```python
from build123d import *

# Parameters (mm, degrees)
SKETCH1_R           = 1.75
BOSS_EXTRUDE1_DEPTH = 5
SKETCH2_R           = 1.75
SKETCH2_R_2         = 6.2
CUT_EXTRUDE1_DEPTH  = 10


with BuildPart() as part:
    # Sketch1 → Boss-Extrude1 (new body)
    # profile 1 of 4: a face of its own
    with BuildSketch(Plane(origin=(0, 0, 0), x_dir=(1, 0, 0), z_dir=(0, 1, 0))):
        Polygon((50, 25), (0, 25), (0, 15), (10, 0), (26, 0), (36, 15), (50, 15), align=None)
        with Locations(Location((13, 5, 0), (0, 0, 270))):
            Circle(SKETCH1_R, mode=Mode.SUBTRACT)
        with Locations(Location((23, 5, 0), (0, 0, 270))):
            Circle(SKETCH1_R, mode=Mode.SUBTRACT)
    # profile 2 of 4: a face of its own
    with BuildSketch(Plane(origin=(0, 0, 0), x_dir=(1, 0, 0), z_dir=(0, 1, 0))):
        Polygon((10, 45), (0, 33.819660113), (0, 25), (50, 25), (50, 35), (36, 35), (26, 45), align=None)
    # profile 3 of 4: a face of its own
    with BuildSketch(Plane(origin=(0, 0, 0), x_dir=(1, 0, 0), z_dir=(0, 1, 0))):
        Polygon((10, 45), (0, 33.819660113), (0, 25), (50, 25), (50, 35), (36, 35), (26, 45), align=None)
    # profile 4 of 4: a face of its own
    with BuildSketch(Plane(origin=(0, 0, 0), x_dir=(1, 0, 0), z_dir=(0, 1, 0))):
        Polygon((10, 45), (0, 33.819660113), (0, 25), (50, 25), (50, 35), (36, 35), (26, 45), align=None)
    extrude(amount=BOSS_EXTRUDE1_DEPTH)

    # Sketch2 → Cut-Extrude1 (cut)
    with BuildSketch(Plane(origin=(0, 0, 0), x_dir=(-1, 0, 0), z_dir=(0, -1, 0))):
        with Locations(Location((-4.8, 24.409830056, 0), (0, 0, 90))):
            Circle(SKETCH2_R)
        with Locations(Location((-32.8, 24.409830056, 0), (0, 0, 90))):
            Circle(SKETCH2_R_2)
    extrude(amount=-CUT_EXTRUDE1_DEPTH, mode=Mode.SUBTRACT)


solid = part.part
```
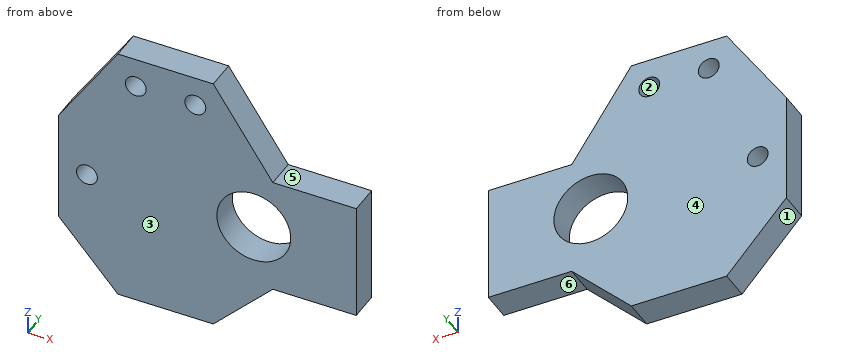
Read the model definition and answer for the solid it produces. Units are mm, in the model's axes. Face numbers are marked on the shaded views. A direction names the side the tool comes from. Coordinates: 2 decimals unless noted, no trailing zeros. Loops run counter-clockwise (first coordinate to the right, second up) from the corner with the lowest first, then second, coordinate; pieces in that order, holes last. Notation, with made-up numbers: (64.5, -39) -> (107.5, -39) arc R25 cw to (107.5, -2) -> close; hole circle Ø7 at (80, -3.5). An arc over 180 degrees is marked (long way). Return JSON: item names as keys, results as strings.
Item 1: For a pull along X with two mould halves and no side action, classify the marked faces 1, 2 and 3 as +X half, -X half, draft (parallel to the pull), parting line (faces both ways), or undercut.
Answers:
{"face 1": "-X half", "face 2": "undercut", "face 3": "draft"}
Item 2: Find section A-A (y = 1.4). Determine the outline of the cut face in (x, z), plus the area to 3 significant figures.
Answers:
{"outline": "(0, -33.82) -> (10, -45) -> (26, -45) -> (36, -35) -> (50, -35) -> (50, -15) -> (36, -15) -> (26, 0) -> (10, 0) -> (0, -15) -> close; hole circle Ø3.5 at (4.8, -24.41); hole circle Ø3.5 at (13, -5); hole circle Ø3.5 at (23, -5); hole circle Ø12.4 at (32.8, -24.41)", "area": "1,490 mm2"}
Item 3: Find section B-B (x = 32.8). Determine the outline of the cut face in (y, z).
Answers:
{"outline": "(0, -38.2) -> (5, -38.2) -> (5, -30.61) -> (0, -30.61) -> close; (0, -18.21) -> (5, -18.21) -> (5, -10.2) -> (0, -10.2) -> close"}
Item 4: Find the intervals of material crossed by probe 1 along X at (y, z) = (4.35, -4); probe 2 along Z at (x, y) = (28.5, 4.35); probe 3 along X at (y, z) = (1.7, -5), in increasing order.
Answers:
{"probe 1": "x = 7.33 to 11.56, 14.44 to 21.56, 24.44 to 28.67", "probe 2": "z = -42.5 to -28.88, -19.94 to -3.75", "probe 3": "x = 6.67 to 11.25, 14.75 to 21.25, 24.75 to 29.33"}
Item 5: Find section C-C (z = -5). Determine the outline of the cut face in (x, y), plus the area to 3 significant figures.
Answers:
{"outline": "(6.67, 0) -> (11.25, 0) -> (11.25, 5) -> (6.67, 5) -> close; (14.75, 0) -> (21.25, 0) -> (21.25, 5) -> (14.75, 5) -> close; (24.75, 0) -> (29.33, 0) -> (29.33, 5) -> (24.75, 5) -> close", "area": "78.3 mm2"}
Item 6: Flat-ended cylindrical pins translate along their axes: P1, Ø5, axis at x = 31, z = -21, coming from the -Y side; P2, Ø2.5, axis at x = 43, y = 1.5, coming from the -Z side. Find the tip coordinate at first contact, or state that the pin passes through.
Answers:
{"P1": "stops at y = 0", "P2": "stops at z = -35"}
Item 7: Find section D-D (x = 23). Determine the outline of the cut face in (y, z), plus the area to 4 significant figures.
Answers:
{"outline": "(0, -45) -> (5, -45) -> (5, -6.75) -> (0, -6.75) -> close; (0, -3.25) -> (5, -3.25) -> (5, 0) -> (0, 0) -> close", "area": "207.5 mm2"}
Item 8: For the marked faces 4, 5 and 6, determine the directions among +Z, -Z, +X, -X, +Y, -Y from which every point of the face is accessible in a straight line to the end or side of a thin tool.
Answers:
{"face 4": "+Z, -Z, +X, -X, +Y", "face 5": "+Z, +X, +Y, -Y", "face 6": "-Z, +X, +Y, -Y"}
